```python
from build123d import *

# Parameters (mm, degrees)
SKETCH_W        = 152.4
SKETCH_H        = 63.5
PAD_DEPTH       = 7.62
SKETCH001_W     = 146.05
SKETCH001_H     = 57.15
PAD001_DEPTH    = 12.7
SKETCH002_W     = 142.367
SKETCH002_H     = 53.975
POCKET_DEPTH    = 9.525
CHAMFER_SIZE    = 12.7
SKETCH003_R     = 18.288
POCKET001_DEPTH = 25.401
SKETCH004_R     = 4.064
PAD002_DEPTH    = 11.0744
SKETCH005_R     = 1.7145
HOLE_DEPTH      = 10.16
HOLE_TIPS_R     = 1.7145
SKETCH006_W     = 2.54
SKETCH006_H     = 53.34
PAD003_DEPTH    = 11.0744
SKETCH008_W     = 66.04
SKETCH008_H     = 27.94
PAD004_DEPTH    = 6.35
SKETCH009_W     = 63.5
SKETCH009_H     = 25.4
POCKET003_DEPTH = 4.445
SKETCH010_W     = 60.452
SKETCH010_H     = 19.6088
POCKET004_DEPTH = 12.701
SKETCH011_W     = 7.62
SKETCH011_H     = 7.62
PAD005_DEPTH    = 12.7
SKETCH012_R     = 2.032
HOLE001_DEPTH   = 11.43
HOLE001_TIPS_R  = 2.032
FILLET_R        = 5.08


with BuildPart() as part:
    # Sketch → Pad (new body)
    with BuildSketch(Plane.XY):
        Rectangle(SKETCH_W, SKETCH_H)
    extrude(amount=PAD_DEPTH)

    # Sketch001 → Pad001 (join)
    with BuildSketch(Plane.XY):
        Rectangle(SKETCH001_W, SKETCH001_H)
    extrude(amount=PAD001_DEPTH)

    # Sketch002 → Pocket (cut)
    with BuildSketch(Plane.XY.offset(12.7)):
        Rectangle(SKETCH002_W, SKETCH002_H)
    extrude(amount=-POCKET_DEPTH, mode=Mode.SUBTRACT)

    # Chamfer
    chamfer_edges = [part.edges().sort_by_distance(p)[0] for p in [
        (-71.1835, 26.9875, 7.9375),
        (-71.1835, -26.9875, 7.9375),
    ]]
    chamfer(chamfer_edges, length=CHAMFER_SIZE)

    # Sketch003 → Pocket001 (cut, through all)
    with BuildSketch(Plane.XY.offset(25.4)):
        with Locations((-44.45, 0)):
            Circle(SKETCH003_R)
    extrude(amount=-POCKET001_DEPTH, mode=Mode.SUBTRACT)

    # Sketch004 → Pad002 (join)
    with BuildSketch(Plane.XY):
        with Locations((-60.6552, -16.1671)):
            Circle(SKETCH004_R)
        with Locations((-28.321, -16.1671)):
            Circle(SKETCH004_R)
        with Locations((-28.321, 16.1671)):
            Circle(SKETCH004_R)
        with Locations((-60.6552, 16.1671)):
            Circle(SKETCH004_R)
    extrude(amount=PAD002_DEPTH)

    # Sketch005 → Hole (cut)
    with BuildSketch(Plane.XY.offset(12.7)):
        with Locations((-60.6552, -16.1671)):
            Circle(SKETCH005_R)
        with Locations((-28.321, -16.1671)):
            Circle(SKETCH005_R)
        with Locations((-28.321, 16.1671)):
            Circle(SKETCH005_R)
        with Locations((-60.6552, 16.1671)):
            Circle(SKETCH005_R)
    extrude(amount=-HOLE_DEPTH, mode=Mode.SUBTRACT)

    # Hole tips → Hole tip 1 section 0
    with BuildSketch(Plane.XY.offset(2.54), mode=Mode.PRIVATE) as hole_tip_1_s0:
        with Locations((-60.6552, -16.1671)):
            Circle(HOLE_TIPS_R)
    loft([hole_tip_1_s0.sketch, Vertex(-60.6552, -16.1671, 1.509824)], mode=Mode.SUBTRACT)

    # Hole tips → Hole tip 2 section 0
    with BuildSketch(Plane.XY.offset(2.54), mode=Mode.PRIVATE) as hole_tip_2_s0:
        with Locations((-28.321, -16.1671)):
            Circle(HOLE_TIPS_R)
    loft([hole_tip_2_s0.sketch, Vertex(-28.321, -16.1671, 1.509824)], mode=Mode.SUBTRACT)

    # Hole tips → Hole tip 3 section 0
    with BuildSketch(Plane.XY.offset(2.54), mode=Mode.PRIVATE) as hole_tip_3_s0:
        with Locations((-28.321, 16.1671)):
            Circle(HOLE_TIPS_R)
    loft([hole_tip_3_s0.sketch, Vertex(-28.321, 16.1671, 1.509824)], mode=Mode.SUBTRACT)

    # Hole tips → Hole tip 4 section 0
    with BuildSketch(Plane.XY.offset(2.54), mode=Mode.PRIVATE) as hole_tip_4_s0:
        with Locations((-60.6552, 16.1671)):
            Circle(HOLE_TIPS_R)
    loft([hole_tip_4_s0.sketch, Vertex(-60.6552, 16.1671, 1.509824)], mode=Mode.SUBTRACT)

    # Sketch006 → Pad003 (join)
    with BuildSketch(Plane.XY):
        with Locations((-24.13, 0)):
            Rectangle(SKETCH006_W, SKETCH006_H)
    extrude(amount=PAD003_DEPTH)

    # Sketch008 → Pad004 (join)
    with BuildSketch(Plane.XY):
        with Locations((14.478, 0)):
            Rectangle(SKETCH008_W, SKETCH008_H)
    extrude(amount=PAD004_DEPTH)

    # Sketch009 → Pocket003 (cut)
    with BuildSketch(Plane.XY.offset(6.35)):
        with Locations((14.478, 0)):
            Rectangle(SKETCH009_W, SKETCH009_H)
    extrude(amount=-POCKET003_DEPTH, mode=Mode.SUBTRACT)

    # Sketch010 → Pocket004 (cut, through all)
    with BuildSketch(Plane.XY.offset(12.7)):
        with Locations((14.097, 0)):
            Rectangle(SKETCH010_W, SKETCH010_H)
    extrude(amount=-POCKET004_DEPTH, mode=Mode.SUBTRACT)

    # Sketch011 → Pad005 (join)
    with BuildSketch(Plane.XY):
        with Locations((51.2826, 23.8125)):
            Rectangle(SKETCH011_W, SKETCH011_H)
        with Locations((51.2826, -23.8125)):
            Rectangle(SKETCH011_W, SKETCH011_H)
    extrude(amount=PAD005_DEPTH)

    # Sketch012 → Hole001 (cut)
    with BuildSketch(Plane.XY.offset(12.7)):
        with Locations((-68.58, 23.876)):
            Circle(SKETCH012_R)
        with Locations((-68.58, -23.876)):
            Circle(SKETCH012_R)
        with Locations((51.054, 23.876)):
            Circle(SKETCH012_R)
        with Locations((51.054, -23.876)):
            Circle(SKETCH012_R)
    extrude(amount=-HOLE001_DEPTH, mode=Mode.SUBTRACT)

    # Hole001 tips → Hole001 tip 1 section 0
    with BuildSketch(Plane.XY.offset(1.27), mode=Mode.PRIVATE) as hole001_tip_1_s0:
        with Locations((-68.58, 23.876)):
            Circle(HOLE001_TIPS_R)
    loft([hole001_tip_1_s0.sketch, Vertex(-68.58, 23.876, 0.049051)], mode=Mode.SUBTRACT)

    # Hole001 tips → Hole001 tip 2 section 0
    with BuildSketch(Plane.XY.offset(1.27), mode=Mode.PRIVATE) as hole001_tip_2_s0:
        with Locations((-68.58, -23.876)):
            Circle(HOLE001_TIPS_R)
    loft([hole001_tip_2_s0.sketch, Vertex(-68.58, -23.876, 0.049051)], mode=Mode.SUBTRACT)

    # Hole001 tips → Hole001 tip 3 section 0
    with BuildSketch(Plane.XY.offset(1.27), mode=Mode.PRIVATE) as hole001_tip_3_s0:
        with Locations((51.054, 23.876)):
            Circle(HOLE001_TIPS_R)
    loft([hole001_tip_3_s0.sketch, Vertex(51.054, 23.876, 0.049051)], mode=Mode.SUBTRACT)

    # Hole001 tips → Hole001 tip 4 section 0
    with BuildSketch(Plane.XY.offset(1.27), mode=Mode.PRIVATE) as hole001_tip_4_s0:
        with Locations((51.054, -23.876)):
            Circle(HOLE001_TIPS_R)
    loft([hole001_tip_4_s0.sketch, Vertex(51.054, -23.876, 0.049051)], mode=Mode.SUBTRACT)

    # Fillet
    fillet_edges = [part.edges().sort_by_distance(p)[0] for p in [
        (-76.2, 31.75, 3.81),
        (0, 31.75, 0),
        (76.2, 31.75, 3.81),
        (-76.2, 0, 0),
        (-76.2, -31.75, 3.81),
        (0, -31.75, 0),
        (76.2, -31.75, 3.81),
        (76.2, 0, 0),
    ]]
    fillet(fillet_edges, radius=FILLET_R)


solid = part.part
```
Model file for the job. Use its own axes, mm. A direction names the side the tool comes from. Give positions to 0.01 mm unless a question says otherwise; leave off trailing zeros.
1) Mould opens along X. For faces 1 (the flat face through (51, 20.002, 8)), 2 (the flat face through (-6, 28, 12.7)), 3 (the flat face through (-76.2, 0, 6)) say: +X half, -X half, draft (parallel to the pull), parting line (faces both ways), or undercut.
2) Pin check, flat tips, straight feed: pin 1 (1.5 mm diameter, centred on x = 14.5, y = 13.5, fed in from +Z); pin 2 (0.6 mm diameter, centred on y = 0.5, z = 1, fed in from -X); pin 3 (1.5 mm diameter, centred on y = 3.5, z = 11, fed in from -X) (3 decimals). Stop position of each tip, or through.
3) Wall check: probe 1 along Y at (x, z) = (33.5, 6.5); probe 2 along X at (y, z) = (18.5, 3.5); probe 3 along Y at (x, z) = (37, 7.75) (1 decimal). Give the ranges that are in metal, low to high.
4) 3-axis set-ups, long thin cutter, end or side, ignore diameter. For faces 4 (the flat face through (-61, 14, 11.074)), 5 (the flat face through (-1, -31.75, 6)): which of +Z, -Z, +X, -X, +Y, -Y reach the whole face in a straight line?
Computed:
1. face 1: undercut
1. face 2: draft
1. face 3: -X half
2. pin 1: stops at z = 6.35
2. pin 2: stops at x = -74.51
2. pin 3: stops at x = -73.025
3. probe 1: y = -31.75 to -26.99, 26.99 to 31.75
3. probe 2: x = -75.95 to -66.97, -63.98 to -57.33, -31.65 to -22.86, 71.18 to 75.95
3. probe 3: y = -28.6 to -27, 27 to 28.6
4. face 4: +Z
4. face 5: +Z, -Z, +X, -X, -Y
